from build123d import *

# Parameters (mm, degrees)
SKETCH1_W                = 40
SKETCH1_H                = 15
BOSS_EXTRUDE1_DEPTH      = 2
SKETCH2_R                = 3.5
CUT_EXTRUDE1_DEPTH       = 2
SKETCH3_W                = 4
SKETCH3_H                = 15
BOSS_EXTRUDE2_DEPTH      = 4
SKETCH4_R                = 0.7
CUT_EXTRUDE2_DEPTH       = 63.0262757
M1_6X0_35_TAPPED_HOLE5_D = 1.25
SKETCH38_R               = 1
BOSS_EXTRUDE4_DEPTH      = 4
M1_6X0_35_TAPPED_HOLE9_D = 1.25
SKETCH41_W               = 4
SKETCH41_H               = 6
CUT_EXTRUDE3_DEPTH       = 10


with BuildPart() as part:
    # Sketch1 → Boss-Extrude1 (new body)
    with BuildSketch(Plane(origin=(0, 0, 0), x_dir=(1, 0, 0), z_dir=(0, 1, 0))):
        with Locations((-39.885381165, 7.155172414)):
            Rectangle(SKETCH1_W, SKETCH1_H)
    extrude(amount=BOSS_EXTRUDE1_DEPTH)

    # Sketch2 → Cut-Extrude1 (cut)
    with BuildSketch(Plane(origin=(0, 2, 0), x_dir=(1, 0, 0), z_dir=(0, 1, 0))):
        with Locations(Location((-39.885381165, 8.155172414, 0), (0, 0, 270))):
            Circle(SKETCH2_R)
    extrude(amount=-CUT_EXTRUDE1_DEPTH, mode=Mode.SUBTRACT)

    # Sketch3 → Boss-Extrude2 (add)
    with BuildSketch(Plane(origin=(0, 2, 0), x_dir=(1, 0, 0), z_dir=(0, 1, 0))):
        with Locations((-57.885381165, 7.155172414)):
            Rectangle(SKETCH3_W, SKETCH3_H)
        with Locations((-21.885381165, 7.155172414)):
            Rectangle(SKETCH3_W, SKETCH3_H)
    extrude(amount=BOSS_EXTRUDE2_DEPTH)

    # Sketch4 → Cut-Extrude2 (cut, through all)
    with BuildSketch(Plane(origin=(0, 0, -14.655172414), x_dir=(-1, 0, 0), z_dir=(0, 0, -1))):
        with Locations((57.885381165, 3)):
            Circle(SKETCH4_R)
        with Locations((21.885381165, 3)):
            Circle(SKETCH4_R)
    extrude(amount=-CUT_EXTRUDE2_DEPTH, mode=Mode.SUBTRACT)

    # M1.6x0.35 Tapped Hole5 (through all)
    with Locations(Plane(origin=(0, 2, 0), x_dir=(1, 0, 0), z_dir=(0, 1, 0))):
        with Locations((-42.385381165, 3.825045395), (-44.885381165, 8.155172414), (-37.337826877, 3.852851279), (-34.885684623, 8.210258577), (-42.385381165, 12.485299433), (-37.385381165, 12.485299433)):
            Hole(M1_6X0_35_TAPPED_HOLE5_D / 2)

    # Sketch38 → Boss-Extrude4 (add)
    with BuildSketch(Plane(origin=(0, 2, 0), x_dir=(1, 0, 0), z_dir=(0, 1, 0))):
        with Locations(Location((-52.385381165, 8.155172414, 0), (0, 0, 270))):
            Circle(SKETCH38_R)
        with Locations(Location((-27.385381165, 8.155172414, 0), (0, 0, 270))):
            Circle(SKETCH38_R)
    extrude(amount=-BOSS_EXTRUDE4_DEPTH)

    # M1.6x0.35 Tapped Hole9 (through all)
    with Locations(Plane(origin=(0, -2, 0), x_dir=(-1, 0, 0), z_dir=(0, -1, 0))):
        with Locations((52.385381165, 8.155172414), (27.385381165, 8.155172414)):
            Hole(M1_6X0_35_TAPPED_HOLE9_D / 2)

    # Sketch41 → Cut-Extrude3 (cut)
    with BuildSketch(Plane(origin=(0, 0, -14.655172414), x_dir=(-1, 0, 0), z_dir=(0, 0, -1))):
        with Locations((57.885381165, 3)):
            Rectangle(SKETCH41_W, SKETCH41_H)
        with Locations((21.885381165, 3)):
            Rectangle(SKETCH41_W, SKETCH41_H)
    extrude(amount=-CUT_EXTRUDE3_DEPTH, mode=Mode.SUBTRACT)


solid = part.part
Design review of the part built by this model. Coordinates are the model's own, in mm. A direction names the side the tool comes from. Give positions to 0.01 mm unless a question says otherwise; leave off trailing zeros. Order: outer loops, then holes, each group sorted by start corner. A loop starts at its lowest first (then second) coordinate and runs counter-clockwise, first axis right, second up.
1. To check wall thickness, follow L1, parallel to X at y = 1.75, z = -8.25; L2, parallel to X at y = 1.25, z = -12.25; L3, parallel to X at y = 2.75, z = -0.25. State the ranges of each line that lie inside material, in increasing order.
Solution:
L1: x = -55.89 to -53, -51.77 to -45.5, -44.27 to -43.38, -36.39 to -35.51, -34.26 to -28, -26.77 to -23.89
L2: x = -55.89 to -42.96, -41.81 to -37.96, -36.81 to -23.89
L3: x = -59.89 to -58.54, -57.23 to -55.89, -23.89 to -22.54, -21.23 to -19.89
2. Tool access review of faces 1 (the flat face through (-22, 4, -4.655)), 2 (the flat face through (-40, 2, -4)), 3 (the flat face through (-58, 6, -2)), 4 (the cylindrical face through (-26.394, -0.986, -8.285)): name each direction out of +Z, -Z, +X, -X, +Y, -Y from which nothing blocks a thin tool from reaching the whole face with its end or side.
Solution:
face 1: -Z, +X, +Y, -Y
face 2: +Z, -Z, +Y
face 3: +Z, -Z, +X, -X, +Y
face 4: -Y
3. Add section D-D, the plane y = 3. State the section outline as (x, z) points.
Solution:
outline: (-59.89, -4.66) - (-58.59, -4.66) - (-58.59, 0.34) - (-59.89, 0.34) - close; (-57.19, -4.66) - (-55.89, -4.66) - (-55.89, 0.34) - (-57.19, 0.34) - close; (-23.89, -4.66) - (-22.59, -4.66) - (-22.59, 0.34) - (-23.89, 0.34) - close; (-21.19, -4.66) - (-19.89, -4.66) - (-19.89, 0.34) - (-21.19, 0.34) - close
4. Add section C-C, the plane z = -11. State the section outline as (x, y) points.
Solution:
outline: (-55.89, 0) - (-41.92, 0) - (-41.92, 2) - (-55.89, 2) - close; (-37.85, 0) - (-23.89, 0) - (-23.89, 2) - (-37.85, 2) - close
5. Mouldability with a two-part tool opening along Z and no side actions: class faces 5 (the cylindrical face through (-34.75, 0.99, -7.6)), 6 (the flat face through (-40, 0, -4)), 7 (the flat face through (-40, 1, -14.655)) as +Z half, -Z half, draft (parallel to the pull), parting line (faces both ways), or undercut.
Solution:
face 5: undercut
face 6: draft
face 7: -Z half
6. Add section A-A, the plane y = 4.75. State the section outline as (x, z) points.
Solution:
outline: (-59.89, -4.66) - (-55.89, -4.66) - (-55.89, 0.34) - (-59.89, 0.34) - close; (-23.89, -4.66) - (-19.89, -4.66) - (-19.89, 0.34) - (-23.89, 0.34) - close
7. For pin 1 Ø8 at (x, z) = (-36, -11) entering from -Y; pin 2 Ø1 at (x, z) = (-48.5, -5) entering from +Y; pin 3 Ø1.8 at (x, y) = (-57.89, 3) entering from -Z, all flat-tipped, find the tip position at first contact; note any pin that passes through.
Solution:
pin 1: stops at y = 0
pin 2: stops at y = 2
pin 3: stops at z = -4.66
8. Add section B-B, the plane x = -42.5. State the section outline as (y, z) points, then the cut area to 3 significant figures.
Solution:
outline: (0, -14.66) - (2, -14.66) - (2, -13.1) - (0, -13.1) - close; (0, -11.87) - (2, -11.87) - (2, -10.48) - (0, -10.48) - close; (0, -5.83) - (2, -5.83) - (2, -4.44) - (0, -4.44) - close; (0, -3.21) - (2, -3.21) - (2, 0.34) - (0, 0.34) - close
area: 15.8 mm2
